Could you check a few things on this model? Use its own coordinates, in mm. Give positions to 0.01 mm unless a question says otherwise; leave off trailing zeros. Write each loop counter-clockwise with the first axis right and the second up, starting at its lowest first coordinate (ties: lowest second). Pieces come first, ordered by that corner, then holes. Notation, with made-up numbers: M 2,57.5 L 33,57.5 A22 cw 33,76.5 Z; hole C 6.5,86.5 d1. An arc over 180 degrees is marked long. Answer as CSV lines item,"result". Start each with the question number.
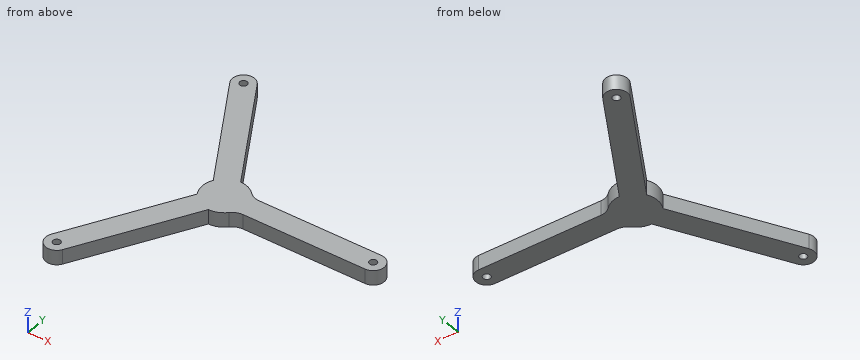
from build123d import *

# Parameters (mm, degrees)
SKETCH1_R           = 2.5
BOSS_EXTRUDE1_DEPTH = 10
FILLET1_R           = 10
CIRPATTERN1_COUNT   = 3


with BuildPart() as part:
    # Sketch1 → Boss-Extrude1 (new body)
    with BuildSketch(Plane.XY):
        with BuildLine():
            Line((12.990381057, -7.5), (100, -7.5))
            ThreePointArc((100, -7.5), (107.5, 0), (100, 7.5))
            Line((100, 7.5), (12.990381057, 7.5))
            ThreePointArc((12.990381057, 7.5), (-15, 0), (12.990381057, -7.5))
        make_face()
        with Locations((100, 0)):
            Circle(SKETCH1_R, mode=Mode.SUBTRACT)
    boss_extrude1 = extrude(amount=BOSS_EXTRUDE1_DEPTH)

    # Fillet1
    fillet1_edges = [part.edges().sort_by_distance(p)[0] for p in [
        (12.990381057, -7.5, 5),
        (12.990381057, 7.5, 5),
    ]]
    fillet(fillet1_edges, radius=FILLET1_R)

    # CirPattern1: Boss-Extrude1 ×3 about axis
    cirpattern1_axis = Axis((0, 0, 0), (0, 0, 1))
    for i in range(1, CIRPATTERN1_COUNT):
        add(boss_extrude1.rotate(cirpattern1_axis, i * 360 / CIRPATTERN1_COUNT))


solid = part.part
1. Will these pins go through, and if not, where does the flat tip stop? P1, Ø6, axis at y = 2.5, z = 5.5, coming from the -X side; P2, Ø5, axis at y = 43.5, z = 5, coming from the -X side; P3, Ø3, axis at x = -7, z = 3, coming from the -Y side.
2. Please list where these lines run through material, in increasing order: line 1 (Y direction, x = 100, z = 7.25); line 2 (Y direction, x = 47, z = 8.25); line 3 (X direction, y = 38, z = 5.5).
3. Imagine slicing it at C-C, the plane x = 83. Please give me the cut outline in (y, z).
4. Imagine slicing it at D-D, the plane y = 70.5. Please give me the cut outline in (x, z).
5. Imagine slicing it at A-A, the plane y = 0. Please give me the cut outline in (x, z), plus the area to 4 significant figures.
6. Imagine slicing it at B-B, the plane z = 2.25. Please give me the cut outline in (x, y), plus the area to 3 significant figures.
Solutions:
1,P1,"x = -15"
1,P2,"x = -35.22"
1,P3,"y = -29.72"
2,line 1,"-7.5 to -2.5, 2.5 to 7.5"
2,line 2,"-7.5 to 7.5"
2,line 3,"-30.6 to -13.28"
3,outline,"M -7.5,0 L 7.5,0 L 7.5,10 L -7.5,10 Z"
4,outline,"M -49.36,0 L -32.04,0 L -32.04,10 L -49.36,10 Z"
5,outline,"M -15,0 L 97.5,0 L 97.5,10 L -15,10 Z; M 102.5,0 L 107.5,0 L 107.5,10 L 102.5,10 Z"
5,area,"1,175 mm²"
6,outline,"M -56.5,-82.85 A7.5 ccw -43.5,-90.35 L 0,-15 A15 ccw 10.71,-10.5 A10 cw 17.85,-7.5 L 100,-7.5 A7.5 ccw 100,7.5 L 17.85,7.5 A10 cw 10.71,10.5 A15 ccw 0,15 L -43.5,90.35 A7.5 ccw -56.5,82.85 L -12.99,7.5 A15 ccw -12.99,-7.5 Z; hole C -50,-86.6 d5; hole C -50,86.6 d5; hole C 100,0 d5"
6,area,"4,770 mm²"
